Source: CAD feature listing. Evaluate the final solid. Frame: model axes, mm. Round coordinates to 2 decimals unless told otherwise and drop trailing zeros. Loops run counter-clockwise (first coordinate to the right, second up) from the corner with the lowest first, then second, coordinate; pieces in that order, holes last.
(1) Section C-C, the plane z = 449.5. Return the cut outline in (x, y), plus the area to 3 significant figures.
(2) Material intervals for probe 1 along Z at (x, y) = (-3.2, -40); probe 2 along Y at (x, z) = (-1.2, 498); probe 3 along Y at (x, z) = (-2.3, 358), sorted ascending.
(3) First-contact query: pin 1 Ø4.5 at (y, z) = (-1.42, 457.75) entering from +X; pin 2 Ø4 at (y, z) = (30.1, 510.77) entering from -X; pin 3 Ø2 at (x, z) = (-2.5, 463) entering from -Y; pin 4 Ø2 at (x, z) = (-1.5, 462) entering from +Y. Flat tips, straight axial feed; report the tip coordinate or a pass-through.
(4) Section B-B, the plane y = 5.5. Return the cut outline in (x, z).
(5) Section A-A, the plane x = -2.4. Count the separate pieces of the cut face and the enclosed holes in it, plus the area to 3 significant figures.
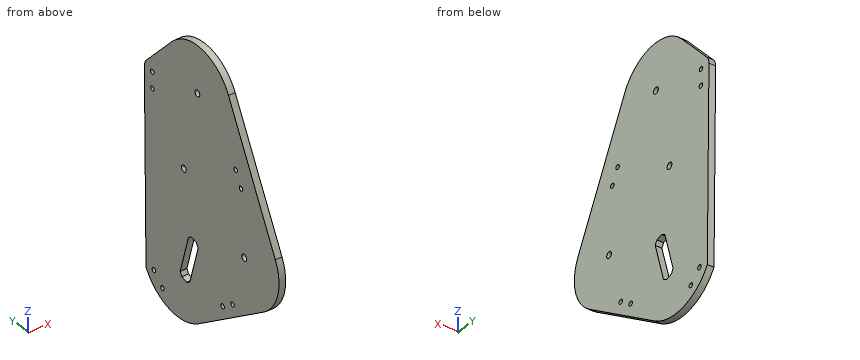
```python
from build123d import *

# Parameters (mm, degrees)
SKETCH4_R           = 1.7272
BOSS_EXTRUDE1_DEPTH = 5
SKETCH6_R           = 2.38125
CUT_EXTRUDE3_DEPTH  = 6


with BuildPart() as part:
    # Sketch4 → Boss-Extrude1 (new body)
    with BuildSketch(Plane(origin=(0, 0, 0), x_dir=(0, 0, -1), z_dir=(1, 0, 0))):
        with BuildLine():
            Line((-510.682190934, 38.038925927), (-365.377526066, 36.419992053))
            ThreePointArc((-365.377526066, 36.419992053), (-347.780080684, 12.728604031), (-353.180701811, -16.284931462))
            Line((-353.180701811, -16.284931462), (-397.273694981, -81.364150349))
            ThreePointArc((-397.273694981, -81.364150349), (-417.278222711, -95.513055214), (-441.64877195, -92.973573308))
            Line((-441.64877195, -92.973573308), (-535.34498696, -46.137884003))
            ThreePointArc((-535.34498696, -46.137884003), (-554.231450435, -19.972248852), (-543.504008498, 10.46228671))
            Line((-543.504008498, 10.46228671), (-516.180391889, 35.910386439))
            ThreePointArc((-516.180391889, 35.910386439), (-513.636251412, 37.504085531), (-510.682190934, 38.038925927))
        make_face()
        with Locations((-485.252549027, -53.289868312)):
            Circle(SKETCH4_R, mode=Mode.SUBTRACT)
        with Locations((-474.518853752, -58.65529334)):
            Circle(SKETCH4_R, mode=Mode.SUBTRACT)
        with Locations((-510.7706223, 30.101918548)):
            Circle(SKETCH4_R, mode=Mode.SUBTRACT)
        with Locations((-498.771367049, 29.968227033)):
            Circle(SKETCH4_R, mode=Mode.SUBTRACT)
        with Locations((-367.666774725, 28.507505411)):
            Circle(SKETCH4_R, mode=Mode.SUBTRACT)
        with Locations((-359.276554144, 19.928216477)):
            Circle(SKETCH4_R, mode=Mode.SUBTRACT)
        with Locations((-385.737171654, -50.185658721)):
            Circle(SKETCH4_R, mode=Mode.SUBTRACT)
        with Locations((-379.006254083, -40.251135649)):
            Circle(SKETCH4_R, mode=Mode.SUBTRACT)
    extrude(amount=-BOSS_EXTRUDE1_DEPTH)

    # Sketch6 → Cut-Extrude3 (cut, through all)
    with BuildSketch(Plane(origin=(0, 0, 0), x_dir=(0, 0, -1), z_dir=(1, 0, 0))):
        with Locations((-519.783421193, -15.006500358)):
            Circle(SKETCH6_R)
        with Locations((-457.75455229, -1.41718755)):
            Circle(SKETCH6_R)
        with Locations((-426.087206182, -61.842189663)):
            Circle(SKETCH6_R)
        Polygon((-410.800244566, -14.012433181), (-407.736158639, -15.718577512), (-378.497536933, -7.395218158), (-376.791392602, -4.331132231), (-378.160423785, 0.478053958), (-381.224509713, 2.184198289), (-410.463131418, -6.139161065), (-412.169275749, -9.203246993), align=None)
    extrude(amount=-CUT_EXTRUDE3_DEPTH, mode=Mode.SUBTRACT)


solid = part.part
```
Output values:
1. outline: (-5, -89.05) - (0, -89.05) - (0, 37.36) - (-5, 37.36) - close
1. area: 632 mm2
2. probe 1: z = 369.25 to 377.3, 380.72 to 544
2. probe 2: y = -64.81 to 28.42, 31.51 to 37.9
2. probe 3: y = -23.4 to 18.76, 21.09 to 30.86
3. pin 1: passes through
3. pin 2: stops at x = -5
3. pin 3: stops at y = -82.8
3. pin 4: stops at y = 37.51
4. outline: (-5, 346.85) - (0, 346.85) - (0, 547.9) - (-5, 547.9) - close
5. separate pieces: 1
5. enclosed holes: 12
5. area: 19,900 mm2
